Work out the finished part from the listing and answer in its coordinate system (mm). Face numbers are marked on the shaded views. A direction names the side the tool comes from. Round coordinates to 2 decimals unless told otherwise and drop trailing zeros. Loops run counter-clockwise (first coordinate to the right, second up) from the corner with the lowest first, then second, coordinate; pieces in that order, holes last.
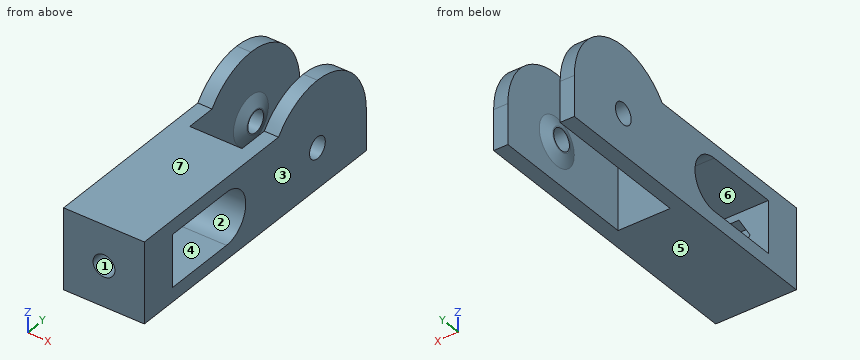
from build123d import *

# Parameters (mm, degrees)
BOSS_EXTRUDE1_DEPTH  = 22.5
CUT_EXTRUDE1_DEPTH   = 70.480213011
SKETCH3_R            = 2.3
CUT_EXTRUDE2_DEPTH   = 8
CUT_EXTRUDE3_DEPTH   = 3
SKETCH5_R            = 5
SKETCH6_R            = 2.5
M4_CLEARANCE_HOLE1_D = 4.5


with BuildPart() as part:
    # Sketch1 → Boss-Extrude1 (new body)
    with BuildSketch(Plane.XY):
        Polygon((0, 0), (17, 0), (17, 63.5), (14, 63.5), (14, 32), (3, 32), (3, 63.5), (0, 63.5), align=None)
    extrude(amount=BOSS_EXTRUDE1_DEPTH)

    # Sketch2 → Cut-Extrude1 (cut, through all)
    with BuildSketch(Plane(origin=(17, 0, 0), x_dir=(0, 0, -1), z_dir=(1, 0, 0))):
        with BuildLine():
            ThreePointArc((-3, 23.5), (-8.5, 29), (-14, 23.5))
            Line((-14, 23.5), (-14, 8))
            Line((-14, 8), (-3, 8))
            Line((-3, 8), (-3, 23.5))
        make_face()
        with BuildLine():
            ThreePointArc((-17, 38.375702269), (-21.049900398, 43.295163177), (-22.5, 49.5))
            Line((-22.5, 49.5), (-22.5, 0))
            Line((-22.5, 0), (-17, 0))
            Line((-17, 0), (-17, 38.375702269))
        make_face()
        with BuildLine():
            Line((-8.5, 63.5), (-22.5, 63.5))
            Line((-22.5, 63.5), (-22.5, 49.5))
            ThreePointArc((-22.5, 49.5), (-18.399494937, 59.399494937), (-8.5, 63.5))
        make_face()
    extrude(amount=-CUT_EXTRUDE1_DEPTH, mode=Mode.SUBTRACT)

    # Sketch3 → Cut-Extrude2 (cut)
    with BuildSketch(Plane.XZ):
        with Locations(Location((8.5, 8.5, 0), (0, 0, 270))):
            Circle(SKETCH3_R)
    extrude(amount=-CUT_EXTRUDE2_DEPTH, mode=Mode.SUBTRACT)

    # Sketch4 → Cut-Extrude3 (cut)
    with BuildSketch(Plane(origin=(0, 8, 0), x_dir=(1, 0, 0), z_dir=(0, 1, 0))):
        Polygon((3.881197846, -8.5), (6.190598923, -12.5), (10.809401077, -12.5), (13.118802154, -8.5), (10.809401077, -4.5), (6.190598923, -4.5), align=None)
    extrude(amount=-CUT_EXTRUDE3_DEPTH, mode=Mode.SUBTRACT)

    # Sketch5 → Loft1 section 0
    with BuildSketch(Plane.ZY.offset(-14)):
        with Locations((8.5, 49.5)):
            Circle(SKETCH5_R)
    # Sketch6 → Loft1 section 1
    with BuildSketch(Plane.ZY.offset(-13)):
        with Locations((8.5, 49.5)):
            Circle(SKETCH6_R)
    loft1 = loft()

    # Mirror1: Loft1 across plane
    add(loft1.mirror(Plane.ZY.offset(-8.5)))

    # M4 Clearance Hole1 (through all)
    with Locations(Plane(origin=(17, 49.5, 8.5), x_dir=(0, 0, 1), z_dir=(1, 0, 0))):
        with Locations((0, 0)):
            Hole(M4_CLEARANCE_HOLE1_D / 2)


solid = part.part
Item 1: Straight lines are drawn through the part: line 1 (Z direction, x = 0.9, y = 49.5); line 2 (Z direction, x = 2.75, y = 17); line 3 (Y direction, x = 0.85, z = 8.5). For each, find the intervals that lie inside material, in ascending order.
Item 2: Section C-C, the plane x = 11.5 is taken. Give the vertices of the cut face in (y, z), plus the area to 3 significant figures.
Item 3: Section A-A, the plane x = 15.5 is taken. Give the vertices of the cut face in (y, z).
Item 4: Section D-D, the plane z = 14.75 is taken. Give the vertices of the cut face in (x, y), plus the area to 3 significant figures.
Item 5: For the marked faces 1, 2 and 3, determine the directions among +Z, -Z, +X, -X, +Y, -Y from which every point of the face is accessible in a straight line to the end or side of a thin tool.
Item 6: Section B-B, the plane y = 6 is taken. Give the vertices of the cut face in (x, z), plus the area to 3 significant figures.
Item 7: Each of these flat-tipped pins is pushed along its axis until it touches: P1, Ø0.9, axis at x = 8, y = 6.5, coming from the +Z side; P2, Ø1, axis at x = 5, z = 4, coming from the +Y side; P3, Ø3, axis at x = 2.5, y = 46, coming from the +Z side. Where does it stop, or does it pass through?
Item 8: Determine the mould class of the marked faces 4, 5, 6 and 7 for opening direction Z: pulls with the +Z half, pulls with the -Z half, needs draft (parallel to the pull), parting line crosses it, or undercut.
Answer below:
1. line 1: z = 0 to 6.25, 10.75 to 22.5
1. line 2: z = 0 to 3, 14 to 17
1. line 3: y = 0 to 8, 29 to 47.25, 51.75 to 63.5
2. outline: (0, 0) - (32, 0) - (32, 17) - (0, 17) - close; hole (5, 5.7) - (8, 5.7) - (8, 3) - (23.5, 3) arc R5.5 ccw to (23.5, 14) - (8, 14) - (8, 11.3) - (5, 11.3) - close
2. area: 309 mm2
3. outline: (0, 0) - (63.5, 0) - (63.5, 8.5) arc R14 ccw to (38.38, 17) - (0, 17) - close; hole (8, 3) - (23.5, 3) arc R5.5 ccw to (23.5, 14) - (8, 14) - close; hole circle Ø4.5 at (49.5, 8.5)
4. outline: (0, 0) - (17, 0) - (17, 62.03) - (14, 62.03) - (14, 32) - (3, 32) - (3, 62.03) - (0, 62.03) - close
4. area: 724 mm2
5. face 1: -Y
5. face 2: +X, -X
5. face 3: +Z, -Z, +X, +Y, -Y
6. outline: (0, 0) - (17, 0) - (17, 17) - (0, 17) - close; hole (3.88, 8.5) - (6.19, 4.5) - (10.81, 4.5) - (13.12, 8.5) - (10.81, 12.5) - (6.19, 12.5) - close
6. area: 234 mm2
7. P1: stops at z = 17
7. P2: stops at y = 32
7. P3: stops at z = 22.36
8. face 4: undercut
8. face 5: pulls with the -Z half
8. face 6: undercut
8. face 7: pulls with the +Z half
